Here's how the part is built. I have some questions about the finished solid (model axes, mm). A direction names the side the tool comes from. Coordinates: 2 decimals unless noted, no trailing zeros. Write each loop counter-clockwise with the first axis right and the second up, starting at its lowest first coordinate (ties: lowest second). Pieces come first, ordered by that corner, then holes. Notation, with made-up numbers: (39, -28) -> (71, -28) arc R27 ccw to (71, -8) -> close; hole circle Ø1 at (-28, 70). An arc over 180 degrees is marked (long way). Put each result on its own line as item: value. Start each with the question number.
Item 1: I want a section at C-C, the plane x = 0. List the corners of the cut face in (y, z) for me, then the cut area to 3 significant figures.
Item 2: I need wall thicknesses on line 1 (Z direction, x = 4, y = 2.5); line 2 (X direction, y = -0.5, z = 2.45); line 3 (Y direction, x = -1.5, z = 0.9). Which ranges of each line are inside material? Lowest first, please. Write a range as [from, to].
Item 3: If we mould it in two halves opening along X, with no side actions, what happens to faces 3 (the face through (0, 2.2, 3)), 4 (the face through (-0.975, 0.165, 0.761)), 5 (the face through (-1.08, -4.88, 0.99)), 6 (the face through (-1, 3, 5))? For each: released by +X, released by -X, zero draft, split by the parting line, or undercut.
Item 4: I want a section at A-A, the plane z = 4.5. List the corners of the cut face in (x, y) for me, then the cut area to 3 significant figures.
Item 5: For pin 1 (1.3 mm diameter, centred on x = 0, y = 0.5, fed in from +Z); pin 2 (1 mm diameter, centred on y = 2, z = 1, fed in from -X); pin 3 (1.5 mm diameter, centred on x = 2, z = 2, fed in from +Y), each with a flat end and sliding along its axis, tell me the tip position at first contact or that it passes through.
Item 6: I want a section at B-B, the plane y = 0. State how many separate pieces and enclosed holes the cut face has, then the cut area to 3 significant figures.
Item 7: On a 3-axis mill with a long thin cutter (end or side, diameter ignored), from which of +Z, -Z, +X, -X, +Y, -Y can I reach the whole of each face in a straight line? I mean faces 1 (the face through (0, -2.2, 3)), 2 (the face through (2.01, -0.21, 0.76)). Say none if no direction works.
from build123d import *

# Parameters (mm, degrees)
SKETCH_R        = 5
PAD_DEPTH       = 2
SKETCH001_R     = 4
PAD001_DEPTH    = 3
POCKET_DEPTH    = 3
SKETCH003_R     = 0.55
POCKET001_DEPTH = 5.001
FILLET_R        = 0.5
FILLET001_R     = 0.5
FILLET002_R     = 0.2


with BuildPart() as part:
    # Sketch → Pad (new body)
    with BuildSketch(Plane.XY):
        Circle(SKETCH_R)
    extrude(amount=PAD_DEPTH)

    # Sketch001 (on Face3 of Pad) → Pad001 (join)
    with BuildSketch(Plane.XY.offset(2)):
        Circle(SKETCH001_R)
    extrude(amount=PAD001_DEPTH)

    # Sketch002 (on Face5 of Pad001) → Pocket (cut)
    with BuildSketch(Plane.XY.offset(5)):
        with BuildLine():
            ThreePointArc((-1, 2.2), (-3.2, 0), (-1, -2.2))
            Line((-1, -2.2), (1, -2.2))
            ThreePointArc((1, -2.2), (3.2, 0), (1, 2.2))
            Line((-1, 2.2), (1, 2.2))
        make_face()
    extrude(amount=-POCKET_DEPTH, mode=Mode.SUBTRACT)

    # Sketch003 (on Face5 of Pocket) → Pocket001 (cut, through all)
    with BuildSketch(Plane.XY.offset(5)):
        with Locations((-1.5, 0)):
            Circle(SKETCH003_R)
        with Locations((1.5, 0)):
            Circle(SKETCH003_R)
    extrude(amount=-POCKET001_DEPTH, mode=Mode.SUBTRACT)

    # Fillet
    fillet_edges = [part.edges().sort_by_distance(p)[0] for p in [
        (-4, 0, 2),
    ]]
    fillet(fillet_edges, radius=FILLET_R)

    # Fillet001
    fillet001_edges = [part.edges().sort_by_distance(p)[0] for p in [
        (-2.05, 0, 2),
        (0.95, 0, 2),
    ]]
    fillet(fillet001_edges, radius=FILLET001_R)

    # Fillet002
    fillet002_edges = [part.edges().sort_by_distance(p)[0] for p in [
        (-4, 0, 5),
        (-3.2, 0, 5),
        (0, -2.2, 5),
        (3.2, 0, 5),
        (0, 2.2, 5),
    ]]
    fillet(fillet002_edges, radius=FILLET002_R)


solid = part.part
Calculated:
1. outline: (-5, 0) -> (5, 0) -> (5, 2) -> (4.5, 2) arc R0.5 cw to (4, 2.5) -> (4, 4.8) arc R0.2 ccw to (3.8, 5) -> (2.4, 5) arc R0.2 ccw to (2.2, 4.8) -> (2.2, 2) -> (-2.2, 2) -> (-2.2, 4.8) arc R0.2 ccw to (-2.4, 5) -> (-3.8, 5) arc R0.2 ccw to (-4, 4.8) -> (-4, 2.5) arc R0.5 cw to (-4.5, 2) -> (-5, 2) -> close
1. area: 30.9 mm2
2. line 1: z = [0, 2]
2. line 2: x = [-3.97, -3.14], [3.14, 3.97]
2. line 3: y = [-4.77, -0.55], [0.55, 4.77]
3. face 3: undercut
3. face 4: undercut
3. face 5: split by the parting line
3. face 6: zero draft
4. outline: circle Ø8 at (0, 0); hole (-1, -2.2) -> (1, -2.2) arc R2.2 ccw to (1, 2.2) -> (-1, 2.2) arc R2.2 ccw to start
4. area: 26.3 mm2
5. pin 1: stops at z = 2
5. pin 2: stops at x = -4.77
5. pin 3: stops at y = 4.84
6. separate pieces: 3
6. enclosed holes: 0
6. area: 20.3 mm2
7. face 1: +Z
7. face 2: +Z, -Z
